The model under review builds one solid part; all positions refer to its coordinate system, in mm. Face numbers are marked on the shaded views. A direction names the side the tool comes from. Coordinates: 2 decimals unless noted, no trailing zeros. Write each loop counter-clockwise with the first axis right and the second up, starting at its lowest first coordinate (ties: lowest second). Pieces come first, ordered by that corner, then holes. Notation, with made-up numbers: (54, -32) - (72, -32) arc R13 ccw to (72, -21) - close; hole circle Ø4 at (-3.5, 13). An arc over 180 degrees is marked (long way). Return JSON: item names as keys, results as strings. Group by question number.
(1) We need section B-B on y = 15.9. State the section outline as (x, z) points (3 decimals), then the cut area to 3 significant figures.
(2) To check wall thickness, follow L1, parallel to X at y = -19.6, z = 20 (3 decimals); L2, parallel to X at y = 15.9, z = 2.75; L3, parallel to Y at x = 19, z = 40. State the ranges of each line that lie inside material, in increasing order. Write a range as from..to.
(3) We need section A-A on z = 5. State the section outline as (x, y) points, then the cut area to 3 significant figures.
(4) Draft analysis for pull direction Y (two halves, no side actions). For the marked faces 1, 2 and 3, state which applies: released by +Y, released by -Y, zero draft, split by the parting line, or undercut.
(5) We need section D-D on z = 53.5. State the section outline as (x, y) points.
(6) Tool access review of the marked faces 4 and 5: name each direction out of +Z, -Z, +X, -X, +Y, -Y from which nothing blocks a thin tool from reaching the whole face with its end or side.
(7) For pin 1 Ø1.1 at (x, z) = (1, 30) entering from +Y; pin 2 Ø5 at (y, z) = (33, 38) entering from -X; pin 3 Ø6 at (y, z) = (22.5, 19.5) entering from +X, all flat-tipped, find the tip position at first contact; note any pin that passes through.
(8) We need section C-C on x = 6. State the section outline as (y, z) points, then the cut area to 3 significant figures.
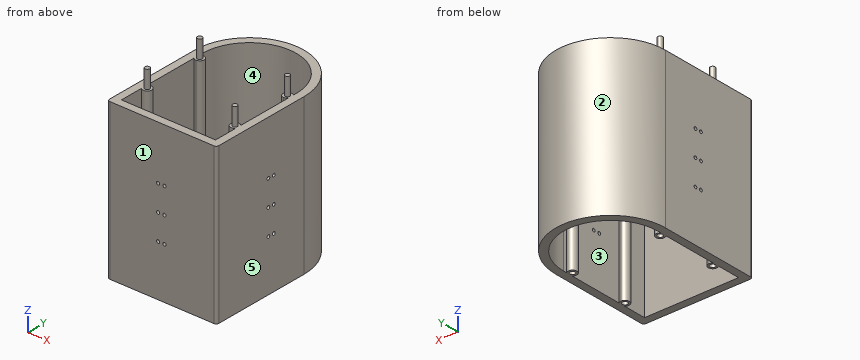
```python
from build123d import *

# Parameters (mm, degrees)
SKETCH2_R           = 1.05
BOSS_EXTRUDE1_DEPTH = 61
BOSS_EXTRUDE2_START = 10
SKETCH2_9_R         = 1.05
BOSS_EXTRUDE2_DEPTH = 58
SKETCH3_R           = 0.625
CUT_EXTRUDE1_DEPTH  = 25
CUT_EXTRUDE2_START  = -25
SKETCH4_R           = 0.625
CUT_EXTRUDE2_DEPTH  = 25
SKETCH5_R           = 0.625
CUT_EXTRUDE3_DEPTH  = 25
CUT_EXTRUDE4_START  = -7
SKETCH6_R           = 1.05
SKETCH6_R_2         = 0.935
CUT_EXTRUDE4_DEPTH  = 7
CUT_EXTRUDE5_START  = -7
SKETCH7_R           = 1.05
SKETCH7_R_2         = 0.935
CUT_EXTRUDE5_DEPTH  = 7
CUT_EXTRUDE6_START  = -7
SKETCH8_R           = 1.05
SKETCH8_R_2         = 0.935
CUT_EXTRUDE6_DEPTH  = 7
CUT_EXTRUDE7_START  = -7
SKETCH9_R           = 1.05
SKETCH9_R_2         = 0.935
CUT_EXTRUDE7_DEPTH  = 7


with BuildPart() as part:
    # Sketch2 → Boss-Extrude1 (new body)
    with BuildSketch(Plane.XY):
        with BuildLine():
            ThreePointArc((21.5, 18.5), (0, 40), (-21.5, 18.5))
            Line((-21.5, 18.5), (-21.5, -20.5))
            ThreePointArc((-21.5, -20.5), (-21.207106781, -21.207106781), (-20.5, -21.5))
            Line((-20.5, -21.5), (20.5, -21.5))
            ThreePointArc((20.5, -21.5), (21.207106781, -21.207106781), (21.5, -20.5))
            Line((21.5, -20.5), (21.5, 18.5))
        make_face()
        with Locations(Location((-17.25, -8.1, 0), (0, 0, 180))):
            Circle(SKETCH2_R, mode=Mode.SUBTRACT)
        with Locations(Location((17.25, -8.1, 0), (0, 0, 180))):
            Circle(SKETCH2_R, mode=Mode.SUBTRACT)
        with Locations(Location((-17.25, 15.9, 0), (0, 0, 180))):
            Circle(SKETCH2_R, mode=Mode.SUBTRACT)
        with BuildLine():
            ThreePointArc((-18.5, -9.324744871), (-15.636648903, -8.77793675), (-17.25, -6.35))
            ThreePointArc((-17.25, -6.35), (-17.92793675, -6.486648903), (-18.5, -6.875255129))
            Line((-18.5, -6.875255129), (-18.5, 14.675255129))
            ThreePointArc((-18.5, 14.675255129), (-17.92793675, 14.286648903), (-17.25, 14.15))
            ThreePointArc((-17.25, 14.15), (-15.636648903, 16.57793675), (-18.5, 17.124744871))
            Line((-18.5, 17.124744871), (-18.5, 18.5))
            ThreePointArc((-18.5, 18.5), (0, 37), (18.5, 18.5))
            Line((18.5, 18.5), (18.5, 17.124744871))
            ThreePointArc((18.5, 17.124744871), (15.636648903, 16.57793675), (17.25, 14.15))
            ThreePointArc((17.25, 14.15), (17.92793675, 14.286648903), (18.5, 14.675255129))
            Line((18.5, 14.675255129), (18.5, -6.875255129))
            ThreePointArc((18.5, -6.875255129), (17.92793675, -6.486648903), (17.25, -6.35))
            ThreePointArc((17.25, -6.35), (15.636648903, -8.77793675), (18.5, -9.324744871))
            Line((18.5, -9.324744871), (18.5, -18.5))
            Line((18.5, -18.5), (-18.5, -18.5))
            Line((-18.5, -18.5), (-18.5, -9.324744871))
        make_face(mode=Mode.SUBTRACT)
        with Locations(Location((17.25, 15.9, 0), (0, 0, 180))):
            Circle(SKETCH2_R, mode=Mode.SUBTRACT)
    extrude(amount=BOSS_EXTRUDE1_DEPTH)

    # Sketch2_9 → Boss-Extrude2 (add)
    with BuildSketch(Plane.XY.offset(BOSS_EXTRUDE2_START)):
        with Locations(Location((-17.25, 15.9, 0), (0, 0, 180))):
            Circle(SKETCH2_9_R)
        with Locations(Location((-17.25, -8.1, 0), (0, 0, 180))):
            Circle(SKETCH2_9_R)
        with Locations(Location((17.25, 15.9, 0), (0, 0, 180))):
            Circle(SKETCH2_9_R)
        with Locations(Location((17.25, -8.1, 0), (0, 0, 180))):
            Circle(SKETCH2_9_R)
    extrude(amount=BOSS_EXTRUDE2_DEPTH)

    # Sketch3 → Cut-Extrude1 (cut)
    with BuildSketch(Plane.ZY.offset(-18.5)):
        with Locations((20, 2.208370448)):
            Circle(SKETCH3_R)
        with Locations((20, 4.708370448)):
            Circle(SKETCH3_R)
        with Locations((30, 2.208370448)):
            Circle(SKETCH3_R)
        with Locations((30, 4.708370448)):
            Circle(SKETCH3_R)
        with Locations((40, 2.208370448)):
            Circle(SKETCH3_R)
        with Locations((40, 4.708370448)):
            Circle(SKETCH3_R)
    extrude(amount=-CUT_EXTRUDE1_DEPTH, mode=Mode.SUBTRACT)

    # Sketch4 → Cut-Extrude2 (cut)
    with BuildSketch(Plane(origin=(-18.5, 0, 0), x_dir=(0, 0, -1), z_dir=(1, 0, 0)).offset(CUT_EXTRUDE2_START)):
        with Locations(Location((-20, 4.708370448, 0), (0, 0, 180))):
            Circle(SKETCH4_R)
        with Locations(Location((-20, 2.208370448, 0), (0, 0, 180))):
            Circle(SKETCH4_R)
        with Locations(Location((-30, 2.208370448, 0), (0, 0, 180))):
            Circle(SKETCH4_R)
        with Locations(Location((-30, 4.708370448, 0), (0, 0, 180))):
            Circle(SKETCH4_R)
        with Locations(Location((-40, 4.708370448, 0), (0, 0, 180))):
            Circle(SKETCH4_R)
        with Locations(Location((-40, 2.208370448, 0), (0, 0, 180))):
            Circle(SKETCH4_R)
    extrude(amount=CUT_EXTRUDE2_DEPTH, mode=Mode.SUBTRACT)

    # Sketch5 → Cut-Extrude3 (cut)
    with BuildSketch(Plane(origin=(0, -18.5, 0), x_dir=(1, 0, 0), z_dir=(0, 1, 0))):
        with Locations(Location((-1.5, -20, 0), (0, 0, 270))):
            Circle(SKETCH5_R)
        with Locations(Location((1, -20, 0), (0, 0, 270))):
            Circle(SKETCH5_R)
        with Locations(Location((-1.5, -30, 0), (0, 0, 270))):
            Circle(SKETCH5_R)
        with Locations(Location((1, -30, 0), (0, 0, 270))):
            Circle(SKETCH5_R)
        with Locations(Location((-1.5, -40, 0), (0, 0, 270))):
            Circle(SKETCH5_R)
        with Locations(Location((1, -40, 0), (0, 0, 270))):
            Circle(SKETCH5_R)
    extrude(amount=-CUT_EXTRUDE3_DEPTH, mode=Mode.SUBTRACT)

    # Sketch6 → Cut-Extrude4 (cut)
    with BuildSketch(Plane.XY.offset(68).offset(CUT_EXTRUDE4_START)):
        with Locations(Location((17.25, 15.9, 0), (0, 0, 180))):
            Circle(SKETCH6_R)
        with Locations((17.25, 15.9)):
            Circle(SKETCH6_R_2, mode=Mode.SUBTRACT)
    extrude(amount=CUT_EXTRUDE4_DEPTH, mode=Mode.SUBTRACT)

    # Sketch7 → Cut-Extrude5 (cut)
    with BuildSketch(Plane.XY.offset(68).offset(CUT_EXTRUDE5_START)):
        with Locations(Location((17.25, -8.1, 0), (0, 0, 180))):
            Circle(SKETCH7_R)
        with Locations((17.25, -8.1)):
            Circle(SKETCH7_R_2, mode=Mode.SUBTRACT)
    extrude(amount=CUT_EXTRUDE5_DEPTH, mode=Mode.SUBTRACT)

    # Sketch8 → Cut-Extrude6 (cut)
    with BuildSketch(Plane.XY.offset(68).offset(CUT_EXTRUDE6_START)):
        with Locations(Location((-17.25, -8.1, 0), (0, 0, 180))):
            Circle(SKETCH8_R)
        with Locations((-17.25, -8.1)):
            Circle(SKETCH8_R_2, mode=Mode.SUBTRACT)
    extrude(amount=CUT_EXTRUDE6_DEPTH, mode=Mode.SUBTRACT)

    # Sketch9 → Cut-Extrude7 (cut)
    with BuildSketch(Plane.XY.offset(68).offset(CUT_EXTRUDE7_START)):
        with Locations(Location((-17.25, 15.9, 0), (0, 0, 180))):
            Circle(SKETCH9_R)
        with Locations((-17.25, 15.9)):
            Circle(SKETCH9_R_2, mode=Mode.SUBTRACT)
    extrude(amount=CUT_EXTRUDE7_DEPTH, mode=Mode.SUBTRACT)


solid = part.part
```
Ans:
{
 "1": {"outline": "(-21.5, 0) - (-18.3, 0) - (-18.3, 10) - (-16.2, 10) - (-16.2, 0) - (-15.5, 0) - (-15.5, 61) - (-16.315, 61) - (-16.315, 68) - (-18.185, 68) - (-18.185, 61) - (-21.5, 61) - close; (15.5, 0) - (16.2, 0) - (16.2, 10) - (18.3, 10) - (18.3, 0) - (21.5, 0) - (21.5, 61) - (18.185, 61) - (18.185, 68) - (16.315, 68) - (16.315, 61) - (15.5, 61) - close", "area": "716 mm²"},
 "2": {"L1": "-21.5..-2.125, -0.875..0.375, 1.625..21.5", "L2": "-21.5..-18.3, -16.2..-15.5, 15.5..16.2, 18.3..21.5", "L3": "-21.5..1.58, 2.83..4.08, 5.33..28.56"},
 "3": {"outline": "(-21.5, -20.5) arc R1 ccw to (-20.5, -21.5) - (20.5, -21.5) arc R1 ccw to (21.5, -20.5) - (21.5, 18.5) arc R21.5 ccw to (-21.5, 18.5) - close; hole (-18.5, -18.5) - (18.5, -18.5) - (18.5, -9.32) arc R1.75 cw (long way) to (18.5, -6.88) - (18.5, 14.68) arc R1.75 cw (long way) to (18.5, 17.12) - (18.5, 18.5) arc R18.5 ccw to (-18.5, 18.5) - (-18.5, 17.12) arc R1.75 cw (long way) to (-18.5, 14.68) - (-18.5, -6.88) arc R1.75 cw (long way) to (-18.5, -9.32) - close; hole circle Ø2.1 at (-17.25, -8.1); hole circle Ø2.1 at (-17.25, 15.9); hole circle Ø2.1 at (17.25, -8.1); hole circle Ø2.1 at (17.25, 15.9)", "area": "560 mm²"},
 "4": {"face 1": "released by -Y", "face 2": "released by +Y", "face 3": "undercut"},
 "5": {"outline": "(-21.5, -20.5) arc R1 ccw to (-20.5, -21.5) - (20.5, -21.5) arc R1 ccw to (21.5, -20.5) - (21.5, 18.5) arc R21.5 ccw to (-21.5, 18.5) - close; hole (-18.5, -18.5) - (18.5, -18.5) - (18.5, -9.32) arc R1.75 cw (long way) to (18.5, -6.88) - (18.5, 14.68) arc R1.75 cw (long way) to (18.5, 17.12) - (18.5, 18.5) arc R18.5 ccw to (-18.5, 18.5) - (-18.5, 17.12) arc R1.75 cw (long way) to (-18.5, 14.68) - (-18.5, -6.88) arc R1.75 cw (long way) to (-18.5, -9.32) - close"},
 "6": {"face 4": "+Z, -Z", "face 5": "+Z, -Z, +X, +Y, -Y"},
 "7": {"pin 1": "y = 40", "pin 2": "x = -17.84", "pin 3": "x = 21.48"},
 "8": {"outline": "(-21.5, 0) - (-18.5, 0) - (-18.5, 61) - (-21.5, 61) - close; (36, 0) - (39.15, 0) - (39.15, 61) - (36, 61) - close", "area": "375 mm²"}
}
